Autodesk Inventor part; units mm, degrees
ref_plane "YZ Plane" through (0, 0, 0) normal (1, 0, 0) x (0, 1, 0)
ref_plane "XZ Plane" through (0, 0, 0) normal (0, 1, 0) x (-1, 0, 0)
ref_plane "XY Plane" through (0, 0, 0) normal (0, 0, 1) x (1, 0, 0)
sketch "Sketch1" plane through (0, 0, 0) normal (0, 0, 1) x (1, 0, 0)
  line L0 (-17.5, 0) -> (17.5, 0) construction
  line L1 (0, -17.5) -> (0, 17.5) construction
  circle A0 centre (0, 0) radius 12.5
  dimension "d0" = 25
extrude "Extrusion1" add sketch "Sketch1" along normal blind 10
sketch "Sketch2" plane through (0, 0, 10) normal (0, 0, 1) x (1, 0, 0)
  circle A0 centre (0, 0) radius 12.5 construction
  circle A1 centre (0, 0) radius 5.5
  dimension "d3" = 11
extrude "Extrusion2" cut sketch "Sketch2" against normal blind 7
sketch "Sketch3" plane through (0, 0, 10) normal (0, 0, 1) x (1, 0, 0)
  circle A0 centre (0, 0) radius 5.5
  circle A1 centre (0, 0) radius 12.5 construction
  line L0 (13.9889, -5.5) -> (-13.9889, -5.5)
  line L1 (-13.9889, -5.5) -> (-13.9889, 5.5)
  line L2 (-13.9889, 5.5) -> (13.9889, 5.5)
  line L3 (13.9889, 5.5) -> (13.9889, -5.5)
  line L4 (13.9889, -5.5) -> (-13.9889, 5.5) construction
  line L5 (-13.9889, -5.5) -> (13.9889, 5.5) construction
  circle A2 centre (0, 0) radius 5.5 construction
extrude "Extrusion3" cut sketch "Sketch3" against normal blind 4.5 contours A0 L2 L3 L0 | A0 L0 L1 L2
ref_plane "Work Plane1" through (0, 12.5, 0) normal (0, -1, 0) x (1, 0, 0)
sketch "Sketch4" plane through (0, 12.5, 0) normal (0, -1, 0) x (1, 0, 0)
  line L0 (-12.5, 0) -> (12.5, 0) construction
  line L1 (-11.225, 10) -> (-11.225, 5.5) construction
  line L2 (-11.225, 5.5) -> (-11.225, 5.5) construction
  line L3 (-11.225, 5.5) -> (-11.225, 10) construction
  line L4 (11.225, 10) -> (-11.225, 10) construction
  line L5 (11.225, 10) -> (11.225, 5.5) construction
  line L6 (11.225, 5.5) -> (11.225, 5.5) construction
  line L7 (11.225, 5.5) -> (11.225, 10) construction
  line L8 (-11.225, 10) -> (11.225, 10) construction
  line L9 (0, -2) -> (0, 12) construction
  circle A0 centre (0, 6) radius 1.6
  point P0 (0, 0)
  dimension "d8" = 3.2
  dimension "d9" = 4
extrude "Extrusion4" cut sketch "Sketch4" along normal through all
Geometry: final body of the model. Coordinates: model frame, mm. A direction names the side the tool comes from. Coordinates: 2 decimals unless noted, no trailing zeros. Loops run counter-clockwise (first coordinate to the right, second up) from the corner with the lowest first, then second, coordinate; pieces in that order, holes last. Notation, with made-up numbers: (0.25, -31.75) -> (31.25, -31.75) arc R22 ccw to (31.25, 3.25) -> close; hole circle Ø1 at (-12.5, 79). An arc over 180 degrees is marked (long way). Use a Markdown table: item, result. Add a question column.
(1) Pin query (flat end, axial travel): pin 1 Ø5 at (x, z) = (4, 8) entering from +Y; pin 2 Ø9 at (x, y) = (-6.5, 0.5) entering from +Z; pin 3 Ø3.5 at (x, y) = (-1.5, 2) entering from +Z. Return the tip coordinate at first contact, or that it passes through.
(2) Section query D-D, the plane z = 6. Return loops of the section in (x, y), plus the area to 3 significant figures.
(3) Section query A-A, the plane x = 0. Return loops of the section in (y, z).
(4) Mould query, pull axis X, two halves, no side actions, for faces 1 (the cylindrical face through (-12.488, -0.55, 4.93)), 2 (the flat face through (0, -5.5, 8)), 3 (the cylindrical face through (-0.35, -8.84, 7.56)). Classes: pulls with the +X half, pulls with the -X half, needs draft (parallel to the pull), parting line crosses it, or undercut.
(5) Line query: line 1 along X through (y, z) = (0, 3.8); line 2 along Z through (x, y) = (0, 10.75). Output: solid intervals per line, ascending.
(6) Section query B-B, the plane z = 8.75. Return loops of the section in (x, y).
(7) Access query for faces 4 (the flat face through (0, 0, 3)), 5 (the flat face through (8, 0, 5.5)), 6 (the flat face through (0, 0, 0)). Directions: +Z, -Z, +X, -X, +Y, -Y. A direction counts if a zero-diameter tool reaches every point of the face in a straight line with its end or side. Return the directions, or none.
(8) Section query C-C, the plane y = 0. Return loops of the section in (x, z), plus the area to 3 significant figures.
Answer:
| question | item | result |
|---|---|---|
| 1 | pin 1 | stops at y = 12.41 |
| 1 | pin 2 | stops at z = 5.5 |
| 1 | pin 3 | stops at z = 3 |
| 2 | outline | (-11.22, -5.5) arc R12.5 ccw to (-1.6, -12.4) -> (-1.6, -5.5) -> close; (-11.22, 5.5) -> (-1.6, 5.5) -> (-1.6, 12.4) arc R12.5 ccw to start; (1.6, -12.4) arc R12.5 ccw to (11.22, -5.5) -> (1.6, -5.5) -> close; (1.6, 5.5) -> (11.22, 5.5) arc R12.5 ccw to (1.6, 12.4) -> close |
| 2 | area | 180 mm^2 |
| 3 | outline | (-12.5, 0) -> (12.5, 0) -> (12.5, 4.4) -> (5.5, 4.4) -> (5.5, 3) -> (-5.5, 3) -> (-5.5, 4.4) -> (-12.5, 4.4) -> close; (-12.5, 7.6) -> (-5.5, 7.6) -> (-5.5, 10) -> (-12.5, 10) -> close; (5.5, 7.6) -> (12.5, 7.6) -> (12.5, 10) -> (5.5, 10) -> close |
| 4 | face 1 | parting line crosses it |
| 4 | face 2 | needs draft |
| 4 | face 3 | undercut |
| 5 | line 1 | x = -12.5 to -5.5, 5.5 to 12.5 |
| 5 | line 2 | z = 0 to 4.4, 7.6 to 10 |
| 6 | outline | (-11.22, -5.5) arc R12.5 ccw to (11.22, -5.5) -> close; (-11.22, 5.5) -> (11.22, 5.5) arc R12.5 ccw to start |
| 7 | face 4 | +Z |
| 7 | face 5 | +Z, +X, -X |
| 7 | face 6 | -Z, +X, -X, +Y, -Y |
| 8 | outline | (-12.5, 0) -> (12.5, 0) -> (12.5, 5.5) -> (5.5, 5.5) -> (5.5, 3) -> (-5.5, 3) -> (-5.5, 5.5) -> (-12.5, 5.5) -> close |
| 8 | area | 110 mm^2 |
